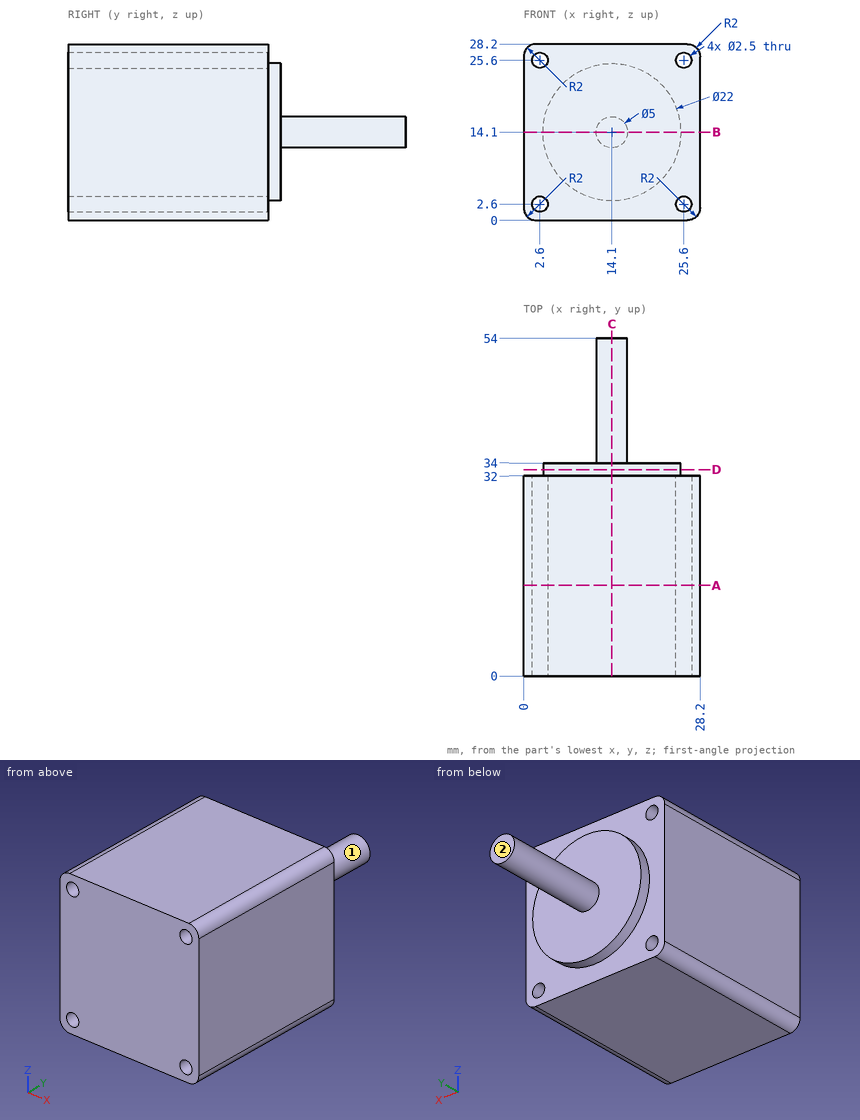
For this review, use the dimensioned drawing (mm, ordinates from the lowest corner) and the shaded views. A direction names the side the tool comes from. Give positions to 0.01 mm unless a question says otherwise; leave off trailing zeros. Write each loop counter-clockwise with the first axis right and the second up, starting at its lowest first coordinate (ties: lowest second). Pieces come first, ordered by that corner, then holes.
(1) Consider section D-D, the plane y = 33. Give the boundary of the cut face in (x, z).
(2) Tool access review of the marked faces 1 and 2: name each direction out of +Z, -Z, +X, -X, +Y, -Y from which nothing blocks a thin tool from reaching the whole face with its end or side.
(3) Consider section B-B, the plane z = 14.1. Give the boundary of the cut face in (x, y), and give its area (3 significant figures).
(4) Consider section C-C, the plane x = 14.1. Give the boundary of the cut face in (y, z).
(5) For P1, Ø1.5, axis at x = 2.6, z = 2.6, coming from the +Y side; P2, Ø6, axis at x = 20, z = 23.5, coming from the +Y side, all flat-tipped, find the tip position at first contact; note any pin that passes through.
(6) Consider section A-A, the plane y = 14.5. Give the boundary of the cut face in (x, z), and give its area (3 significant figures).
(7) To check wall thickness, follow L1, parallel to Z at x = 2.6, y = 25; L2, parallel to Z at x = 3.25, y = 7. State the ranges of each line that lie inside material, in increasing order.
Returned:
1. outline: circle Ø22 at (14.1, 14.1)
2. face 1: +Y
2. face 2: +Z, -Z, +X, -X, +Y
3. outline: (0, 0) - (28.2, 0) - (28.2, 32) - (25.1, 32) - (25.1, 34) - (16.6, 34) - (16.6, 54) - (11.6, 54) - (11.6, 34) - (3.1, 34) - (3.1, 32) - (0, 32) - close
3. area: 1,050 mm2
4. outline: (0, 0) - (32, 0) - (32, 3.1) - (34, 3.1) - (34, 11.6) - (54, 11.6) - (54, 16.6) - (34, 16.6) - (34, 25.1) - (32, 25.1) - (32, 28.2) - (0, 28.2) - close
5. P1: passes through
5. P2: stops at y = 34
6. outline: (0, 2) arc R2 ccw to (2, 0) - (26.2, 0) arc R2 ccw to (28.2, 2) - (28.2, 26.2) arc R2 ccw to (26.2, 28.2) - (2, 28.2) arc R2 ccw to (0, 26.2) - close; hole circle Ø2.5 at (2.6, 2.6); hole circle Ø2.5 at (2.6, 25.6); hole circle Ø2.5 at (25.6, 2.6); hole circle Ø2.5 at (25.6, 25.6)
6. area: 772 mm2
7. L1: z = 0 to 1.35, 3.85 to 24.35, 26.85 to 28.2
7. L2: z = 0 to 1.53, 3.67 to 24.53, 26.67 to 28.2
